Could you check a few things on this model? Use its own coordinates, in mm. Coordinates: 2 decimals unless noted, no trailing zeros. Write each loop counter-clockwise with the first axis right and the second up, starting at its lowest first coordinate (ties: lowest second). Pieces come first, ordered by that corner, then holes.
```python
from build123d import *

# Parameters (mm, degrees)
SKETCH_1_W          = 127.5
SKETCH_1_H          = 70
SKETCH_1_R          = 1.6
EXTRUDE_1_DEPTH     = 1
SKETCH_2_W          = 127.5
SKETCH_2_H          = 3
CUT_EXTRUDE_1_DEPTH = 10
SKETCH_3_W          = 22
SKETCH_3_H          = 67
CUT_EXTRUDE_2_DEPTH = 10
SKETCH_4_W          = 3
SKETCH_4_H          = 67
EXTRUDE_3_DEPTH     = 1
SKETCH_5_W          = 30
SKETCH_5_H          = 6
CUT_EXTRUDE_3_DEPTH = 5
FILLET_1_R          = 1
FILLET_2_R          = 2
SKETCH_6_R          = 10.184947092
CUT_EXTRUDE_4_DEPTH = 5


with BuildPart() as part:
    # 草图1 → 凸台-拉伸1 (new body)
    with BuildSketch(Plane.XY):
        Rectangle(SKETCH_1_W, SKETCH_1_H)
        with Locations((-7, 22.9)):
            Circle(SKETCH_1_R, mode=Mode.SUBTRACT)
        with Locations((7, 22.9)):
            Circle(SKETCH_1_R, mode=Mode.SUBTRACT)
    extrude(amount=EXTRUDE_1_DEPTH)

    # 草图2 → 切除-拉伸1 (cut)
    with BuildSketch(Plane.XY.offset(1)):
        with Locations((0, 33.5)):
            Rectangle(SKETCH_2_W, SKETCH_2_H)
    extrude(amount=-CUT_EXTRUDE_1_DEPTH, mode=Mode.SUBTRACT)

    # 草图3 → 切除-拉伸2 (cut)
    with BuildSketch(Plane.XY.offset(1)):
        with Locations((52.75, -1.5)):
            Rectangle(SKETCH_3_W, SKETCH_3_H)
    extrude(amount=-CUT_EXTRUDE_2_DEPTH, mode=Mode.SUBTRACT)

    # 草图4 → 凸台-拉伸3 (add)
    with BuildSketch(Plane.XY.offset(1)):
        with Locations((-65.25, -1.5)):
            Rectangle(SKETCH_4_W, SKETCH_4_H)
    extrude(amount=-EXTRUDE_3_DEPTH)

    # 草图5 → 切除-拉伸3 (cut, symmetric)
    with BuildSketch(Plane.XY.offset(1)):
        with Locations((0, 32)):
            Rectangle(SKETCH_5_W, SKETCH_5_H)
    extrude(amount=CUT_EXTRUDE_3_DEPTH, both=True, mode=Mode.SUBTRACT)

    # 圆角1
    fillet_1_edges = [part.edges().sort_by_distance(p)[0] for p in [
        (-15, 32, 0.5),
        (15, 32, 0.5),
        (15, 29, 0.5),
        (-15, 29, 0.5),
    ]]
    fillet(fillet_1_edges, radius=FILLET_1_R)

    # 圆角2
    fillet_2_edges = [part.edges().sort_by_distance(p)[0] for p in [
        (41.75, 32, 0.5),
        (41.75, -35, 0.5),
        (-66.75, -35, 0.5),
        (-66.75, 32, 0.5),
    ]]
    fillet(fillet_2_edges, radius=FILLET_2_R)

    # 草图6 → 切除-拉伸4 (cut, symmetric)
    with BuildSketch(Plane(origin=(0, 0, 0), x_dir=(-1, 0, 0), z_dir=(0, 0, -1))):
        with Locations((-9.42, -8.6)):
            Circle(SKETCH_6_R)
        with BuildLine():
            Line((12.759998774, -12.590828373), (12.760187446, -4.590023504))
            add(Edge.make_bspline(
                [(12.760187446, -4.590023504), (12.76034149, -4.131184745), (12.371605061, -3.175167995), (10.96226041, -2.598669542), (9.551855004, -3.173570847), (9.161664376, -4.130045812), (9.161317678, -4.589244926)],
                knots=[0.000124436, 0.000124436, 0.000124436, 0.000124436, 0.250093327, 0.500062218, 0.750031109, 1, 1, 1, 1], degree=3))
            Line((9.161317678, -4.589244926), (9.160940723, -12.589969013))
            add(Edge.make_bspline(
                [(9.160940723, -12.589969013), (9.16093388, -13.04878603), (9.54993428, -14.004593398), (10.95932287, -14.580864951), (12.369900224, -14.00523711), (12.759249328, -13.049723173), (12.759998774, -12.590828373)],
                knots=[-6.415e-06, -6.415e-06, -6.415e-06, -6.415e-06, 0.250075228, 0.50015687, 0.750238513, 1.000320156, 1.000320156, 1.000320156, 1.000320156], degree=3))
        make_face()
        with BuildLine():
            Line((22.409427896, -12.590000012), (22.409427896, -4.589999921))
            ThreePointArc((22.409427896, -4.589999921), (20.60943071, -2.790002734), (18.809433524, -4.589999921))
            Line((18.809433524, -4.589999921), (18.809433524, -12.590000012))
            ThreePointArc((18.809433524, -12.590000012), (20.60943071, -14.389997198), (22.409427896, -12.590000012))
        make_face()
        with BuildLine():
            Line((32.059432501, -12.590000012), (32.059432501, -4.589999921))
            ThreePointArc((32.059432501, -4.589999921), (30.259435314, -2.790002734), (28.459438128, -4.589999921))
            Line((28.459438128, -4.589999921), (28.459438128, -12.590000012))
            ThreePointArc((28.459438128, -12.590000012), (30.259435314, -14.389997198), (32.059432501, -12.590000012))
        make_face()
        with BuildLine():
            Line((41.709430966, -12.590000012), (41.709430966, -4.589999921))
            ThreePointArc((41.709430966, -4.589999921), (39.90943378, -2.790002734), (38.109436593, -4.589999921))
            Line((38.109436593, -4.589999921), (38.109436593, -12.590000012))
            ThreePointArc((38.109436593, -12.590000012), (39.90943378, -14.389997198), (41.709430966, -12.590000012))
        make_face()
    extrude(amount=CUT_EXTRUDE_4_DEPTH, both=True, mode=Mode.SUBTRACT)


solid = part.part
```
1. Please list where these lines run through material, in increasing order: line 1 along Y through (x, z) = (7, 0.55); line 2 along Y through (x, z) = (-7, 0.65); line 3 along X through (y, z) = (-3, 0.65).
Verdict:
line 1: y = -35 to -18.49, 1.29 to 21.3, 24.5 to 29
line 2: y = -35 to 21.3, 24.5 to 29
line 3: x = -66.75 to -40.75, -39.07 to -31.1, -29.42 to -21.45, -19.77 to -11.8, -10.12 to 0.91, 17.93 to 41.75
2. I want a section at A-A on x = -7. Please give me the cut outline in (y, z), plus the area to 3 significant figures.
Verdict:
outline: (-35, 0) - (21.3, 0) - (21.3, 1) - (-35, 1) - close; (24.5, 0) - (29, 0) - (29, 1) - (24.5, 1) - close
area: 60.8 mm2
3. I want a section at C-C on y = -10.5. Please give me the cut outline in (x, z).
Verdict:
outline: (-66.75, 0) - (-41.71, 0) - (-41.71, 1) - (-66.75, 1) - close; (-38.11, 0) - (-32.06, 0) - (-32.06, 1) - (-38.11, 1) - close; (-28.46, 0) - (-22.41, 0) - (-22.41, 1) - (-28.46, 1) - close; (-18.81, 0) - (-12.76, 0) - (-12.76, 1) - (-18.81, 1) - close; (-9.16, 0) - (-0.59, 0) - (-0.59, 1) - (-9.16, 1) - close; (19.43, 0) - (41.75, 0) - (41.75, 1) - (19.43, 1) - close
4. I want a section at D-D on x = 7. Please give me the cut outline in (y, z), plus the area to 3 significant figures.
Verdict:
outline: (-35, 0) - (-18.49, 0) - (-18.49, 1) - (-35, 1) - close; (1.29, 0) - (21.3, 0) - (21.3, 1) - (1.29, 1) - close; (24.5, 0) - (29, 0) - (29, 1) - (24.5, 1) - close
area: 41.0 mm2
5. If we mould it in two halves opening along Y, with no side actions, what happens to faces 1 (the face through (-8.27, 21.93, 0.49)), 2 (the face through (41.18, 31.4, 0.49)), 3 (the face through (-66.18, -34.4, 0.49)), 4 (the face through (19.595, -8.152, 0.493))? For each: pulls with the +Y half, pulls with the -Y half, needs draft (parallel to the pull), parting line crosses it, or undercut.
Verdict:
face 1: undercut
face 2: pulls with the +Y half
face 3: pulls with the -Y half
face 4: undercut
6. For pin 1 (0.5 mm diameter, centred on y = 30.5, z = 0.5, fed in from +X); pin 2 (12 mm diameter, centred on x = 9.42, y = -8.6, fed in from +Z), each with a flat end and sliding along its axis, tell me the tip position at first contact or that it passes through.
Verdict:
pin 1: stops at x = 41.73
pin 2: passes through
7. I want a section at B-B on y = 22.9. Please give me the cut outline in (x, z), plus the area to 3 significant figures.
Verdict:
outline: (-66.75, 0) - (-8.6, 0) - (-8.6, 1) - (-66.75, 1) - close; (-5.4, 0) - (5.4, 0) - (5.4, 1) - (-5.4, 1) - close; (8.6, 0) - (41.75, 0) - (41.75, 1) - (8.6, 1) - close
area: 102 mm2
